Can you work these out from the drawing? Everything is in mm from the part's minimum corner. A direction names the side the tool comes from. Give positions to 0.01 mm unless a question says otherwise; leave off trailing zeros. Loops run counter-clockwise (first coordinate to the right, second up) from the corner with the lowest first, then second, coordinate; pieces in that order, holes last. Notation, with made-up numbers: (10.25, 76.25) - (35.25, 76.25) arc R9 cw to (35.25, 87.25) - close; hole circle Ø2 at (55, 53.25). An arc over 180 degrees is marked (long way). One line per item, written item: value. Start each with the question number.
Q1. If I drill on line 1 (X direction, y = 27.85, z = 5.05); line 2 (X direction, y = 37, z = 9); line 3 (Y direction, x = 10.5, z = 8), over which ranges is the centre line in solid material (lowest first)? Write a range as from..to.
Q2. I'm going to push flat-ended pins straight in: P1, Ø5, axis at x = 1.65, z = 5.05, coming from the -Y side; P2, Ø1.5, axis at x = 31, z = 4.5, coming from the +Y side; P3, Ø1, axis at x = 33, y = 32, coming from the -Z side; P4, Ø2.5, axis at x = 51.15, z = 15.05, coming from the -Y side. Where does each tip first touch, or does it pass through?
Q3. For the marked faces 1, 2 and 3, which set-ups out of +Z, -Z, +X, -X, +Y, -Y let a thin tool reach every point of the face, with its end or its side?
Q4. I want a section at C-C (x = 39.8). Please give me the cut outline in (y, z).
Q5. I want a section at D-D (y = 36.5). Please give me the cut outline in (x, z).
Q6. I want a section at A-A (z = 5.05). Please give me the cut outline in (x, y), then the cut area to 3 significant figures.
Q7. If we mould it in two halves opening along Z, with no side actions, what happens to the marked faces 4, 5 and 6? For each: released by +Z, released by -Z, zero draft, split by the parting line, or undercut.
Q8. I want a section at B-B (x = 1.65). Please give me the cut outline in (y, z), then the cut area to 3 significant figures.
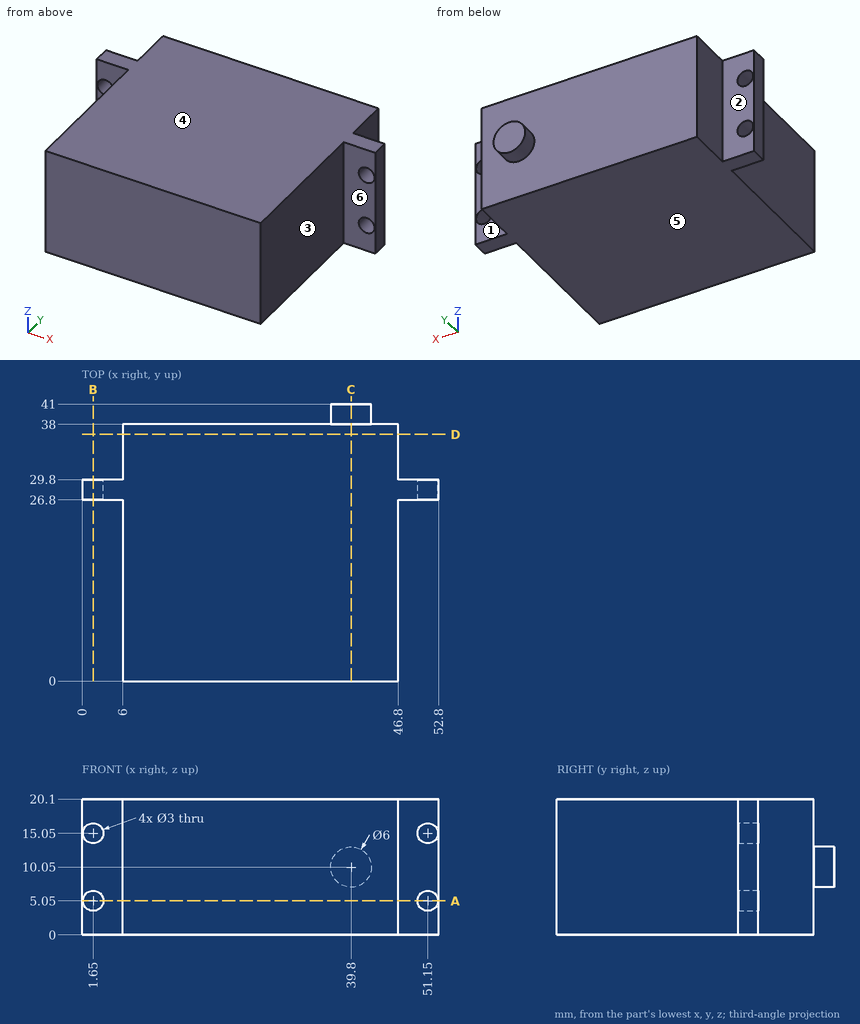
Worked answers:
1. line 1: x = 0..0.15, 3.15..49.65, 52.65..52.8
1. line 2: x = 6..46.8
1. line 3: y = 0..38
2. P1: stops at y = 26.8
2. P2: stops at y = 38
2. P3: stops at z = 0
2. P4: passes through
3. face 1: +Z, -Z, +X, +Y
3. face 2: +Z, -Z, -X, +Y
3. face 3: +Z, -Z, +X, -Y
4. outline: (0, 0) - (38, 0) - (38, 7.05) - (41, 7.05) - (41, 13.05) - (38, 13.05) - (38, 20.1) - (0, 20.1) - close
5. outline: (6, 0) - (46.8, 0) - (46.8, 20.1) - (6, 20.1) - close
6. outline: (0, 26.8) - (0.15, 26.8) - (0.15, 29.8) - (0, 29.8) - close; (3.15, 26.8) - (6, 26.8) - (6, 0) - (46.8, 0) - (46.8, 26.8) - (49.65, 26.8) - (49.65, 29.8) - (46.8, 29.8) - (46.8, 38) - (6, 38) - (6, 29.8) - (3.15, 29.8) - close; (52.65, 26.8) - (52.8, 26.8) - (52.8, 29.8) - (52.65, 29.8) - close
6. area: 1,570 mm²
7. face 4: released by +Z
7. face 5: released by -Z
7. face 6: zero draft
8. outline: (26.8, 0) - (29.8, 0) - (29.8, 3.55) - (26.8, 3.55) - close; (26.8, 6.55) - (29.8, 6.55) - (29.8, 13.55) - (26.8, 13.55) - close; (26.8, 16.55) - (29.8, 16.55) - (29.8, 20.1) - (26.8, 20.1) - close
8. area: 42.3 mm²
